Autodesk Inventor part; units mm, degrees
ref_plane "YZ Plane" through (0, 0, 0) normal (1, 0, 0) x (0, 1, 0)
ref_plane "XZ Plane" through (0, 0, 0) normal (0, 1, 0) x (-1, 0, 0)
ref_plane "XY Plane" through (0, 0, 0) normal (0, 0, 1) x (1, 0, 0)
sketch "Sketch1" plane through (0, 0, 0) normal (0, 0, 1) x (1, 0, 0)
  line L0 (0, 0) -> (15.24, 0)
  line L1 (15.24, 0) -> (15.24, -15.24)
  line L2 (15.24, -15.24) -> (0, -15.24)
  line L3 (0, -15.24) -> (0, 0)
  dimension "d0" = 15.24
  dimension "d1" = 15.24
extrude "Extrusion1" add sketch "Sketch1" along normal blind 1.016
sketch "Sketch2" plane through (0, 0, 1.016) normal (0, 0, 1) x (1, 0, 0)
  line L0 (15.24, 0) -> (0, 0)
  line L1 (0, 0) -> (0, -15.24)
  line L2 (15.24, -15.24) -> (15.24, 0)
  circle A0 centre (13.97, -1.27) radius 0.381
  circle A1 centre (13.97, -3.81) radius 0.381
  circle A2 centre (13.97, -6.35) radius 0.381
  circle A3 centre (13.97, -8.89) radius 0.381
  circle A4 centre (13.97, -11.43) radius 0.381
  circle A5 centre (13.97, -13.97) radius 0.381
  circle A6 centre (1.27, -1.27) radius 0.381
  circle A7 centre (1.27, -3.81) radius 0.381
  circle A8 centre (1.27, -6.35) radius 0.381
  circle A9 centre (1.27, -8.89) radius 0.381
  circle A10 centre (1.27, -11.43) radius 0.381
  circle A11 centre (1.27, -13.97) radius 0.381
  dimension "d4" = 0.762
  dimension "d6" = 1.27
  dimension "d7" = 1.27
  dimension "d10" = 2.54
  dimension "d17" = 12.7
extrude "Extrusion2" cut sketch "Sketch2" against normal blind 1.27
properties part number "Board" material "Thermoplastic Resin"
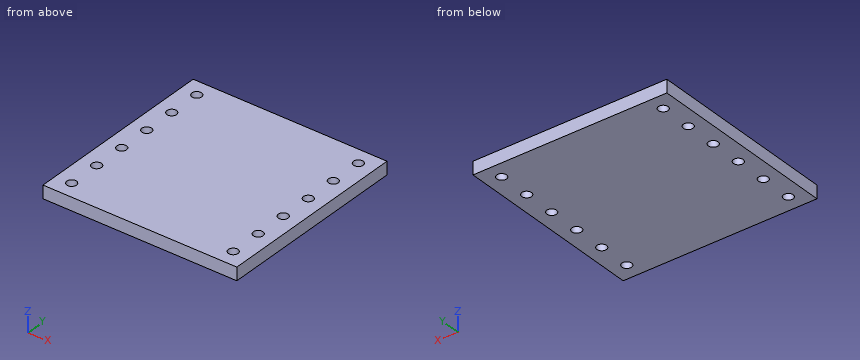
Model file for the job. Use its own axes, mm. Give positions to 0.01 mm unless a question says otherwise; leave off trailing zeros. Order: outer loops, then holes, each group sorted by start corner. A loop starts at its lowest first (then second) coordinate and runs counter-clockwise, first axis right, second up. Notation, with made-up numbers: (82, -15.75) - (113, -15.75) arc R17 ccw to (113, 9.25) - close; hole circle Ø6 at (-27, 49). An arc over 180 degrees is marked (long way). One line per item, written item: value.
Item 1: Slice it at A-A (x = 1.27). List the corners of the cut face in (y, z), then the cut area to 3 significant figures.
Response values:
outline: (-15.24, 0) - (-14.35, 0) - (-14.35, 1.02) - (-15.24, 1.02) - close; (-13.59, 0) - (-11.81, 0) - (-11.81, 1.02) - (-13.59, 1.02) - close; (-11.05, 0) - (-9.27, 0) - (-9.27, 1.02) - (-11.05, 1.02) - close; (-8.51, 0) - (-6.73, 0) - (-6.73, 1.02) - (-8.51, 1.02) - close; (-5.97, 0) - (-4.19, 0) - (-4.19, 1.02) - (-5.97, 1.02) - close; (-3.43, 0) - (-1.65, 0) - (-1.65, 1.02) - (-3.43, 1.02) - close; (-0.89, 0) - (0, 0) - (0, 1.02) - (-0.89, 1.02) - close
area: 10.8 mm2
Item 2: Wall check: line 1 (X direction, y = -1.25, z = 0.6); line 2 (X direction, y = -11.5, z = 0.4). Give the ranges that are in metal, low to high.
Response values:
line 1: 0 to 0.89, 1.65 to 13.59, 14.35 to 15.24
line 2: 0 to 0.9, 1.64 to 13.6, 14.34 to 15.24
Item 3: Slice it at B-B (y = -1.27). List the corners of the cut face in (x, z), then the cut area to 3 significant figures.
Response values:
outline: (0, 0) - (0.89, 0) - (0.89, 1.02) - (0, 1.02) - close; (1.65, 0) - (13.59, 0) - (13.59, 1.02) - (1.65, 1.02) - close; (14.35, 0) - (15.24, 0) - (15.24, 1.02) - (14.35, 1.02) - close
area: 13.9 mm2
